from build123d import *

# Parameters (mm, degrees)
PAD_DEPTH          = 30
SKETCH001_R        = 1.698779
SKETCH001_R_2      = 1.697275
POCKET_DEPTH       = 137.607308
POCKET001_DEPTH    = 3.3
POCKET001_FACE8_W  = 30
POCKET001_FACE8_H  = 12.999695
POCKET001_FACE8_R  = 1.698779
POCKET002_DEPTH    = 0.2
POCKET002_FACE11_W = 30
POCKET002_FACE11_H = 13.000122
POCKET002_FACE11_R = 1.698779
POCKET003_DEPTH    = 0.2
POCKET003_FACE16_W = 30
POCKET003_FACE16_H = 13.005555
POCKET003_FACE16_R = 1.697275
POCKET004_DEPTH    = 0.2
POCKET004_FACE19_W = 30
POCKET004_FACE19_H = 13.004761
POCKET004_FACE19_R = 1.697275
POCKET005_DEPTH    = 0.2


with BuildPart() as part:
    # Sketch → Pad (new body)
    with BuildSketch(Plane.XZ.offset(-204.7)):
        Polygon((442.140533, 170.606308), (570.199951, 170.606308), (570.199951, 160.446457), (557.19519, 160.446457), (557.19519, 144.454102), (570.200745, 144.454102), (570.200745, 134.453659), (442.140106, 134.453659), (442.140106, 144.601944), (455.140228, 144.601944), (455.140228, 160.599991), (442.140533, 160.599991), align=None)
    extrude(amount=-PAD_DEPTH)

    # Sketch001 → Pocket (cut, through all)
    with BuildSketch(Plane.XY.offset(33)):
        with Locations((449.144109, 219.697878)):
            Circle(SKETCH001_R)
        with Locations((563.197394, 219.696552)):
            Circle(SKETCH001_R_2)
    extrude(amount=POCKET_DEPTH, mode=Mode.SUBTRACT)

    # Sketch002 → Pocket001 (cut)
    with BuildSketch(Plane.XY.offset(134.45)):
        Polygon((447.4586694554, 222.4277322113), (445.9354318133, 219.6021619882), (447.6208285856, 216.8702143825), (450.829463, 216.963837), (452.3527006421, 219.7894072231), (450.6673038698, 222.5213548287), align=None)
        Polygon((561.3429027745, 222.3136473905), (560.000239016, 219.3979392379), (561.8539844669, 216.7773042379), (565.0503936764, 217.0723773905), (566.393057435, 219.9880855431), (564.539311984, 222.6087205431), align=None)
    extrude(amount=POCKET001_DEPTH, mode=Mode.SUBTRACT)

    # Pocket001 Face8 → Pocket002 (cut)
    with BuildSketch(Plane(origin=(448.6283915528, 219.7000505045, 160.599991), x_dir=(0, -1, 0), z_dir=(0, 0, -1))):
        with Locations((5.05045e-05, -0.0119889472)):
            Rectangle(POCKET001_FACE8_W, POCKET001_FACE8_H)
        with Locations((0.0021725045, -0.5157174472)):
            Circle(POCKET001_FACE8_R, mode=Mode.SUBTRACT)
    extrude(amount=-POCKET002_DEPTH, mode=Mode.SUBTRACT)

    # Pocket002 Face11 → Pocket003 (cut)
    with BuildSketch(Plane(origin=(448.6281733748, 219.7000505028, 144.601944), x_dir=(0, 1, 0), z_dir=(0, 0, 1))):
        with Locations((-5.05028e-05, -0.0119936252)):
            Rectangle(POCKET002_FACE11_W, POCKET002_FACE11_H)
        with Locations((-0.0021725028, -0.5159356252)):
            Circle(POCKET002_FACE11_R, mode=Mode.SUBTRACT)
    extrude(amount=-POCKET003_DEPTH, mode=Mode.SUBTRACT)

    # Pocket003 Face16 → Pocket004 (cut)
    with BuildSketch(Plane(origin=(563.709854284, 219.7000818773, 144.454102), x_dir=(0, 1, 0), z_dir=(0, 0, 1))):
        with Locations((-8.18773e-05, 0.011886784)):
            Rectangle(POCKET003_FACE16_W, POCKET003_FACE16_H)
        with Locations((-0.0035298773, 0.512460284)):
            Circle(POCKET003_FACE16_R, mode=Mode.SUBTRACT)
    extrude(amount=-POCKET004_DEPTH, mode=Mode.SUBTRACT)

    # Pocket004 Face19 → Pocket005 (cut)
    with BuildSketch(Plane(origin=(563.7094485991, 219.7000818825, 160.446457), x_dir=(0, -1, 0), z_dir=(0, 0, -1))):
        with Locations((8.18825e-05, 0.0118780991)):
            Rectangle(POCKET004_FACE19_W, POCKET004_FACE19_H)
        with Locations((0.0035298825, 0.5120545991)):
            Circle(POCKET004_FACE19_R, mode=Mode.SUBTRACT)
    extrude(amount=-POCKET005_DEPTH, mode=Mode.SUBTRACT)


solid = part.part
Could you check a few things on this model? Use its own coordinates, in mm. A direction names the side the tool comes from. Give positions to 0.01 mm unless a question says otherwise; leave off trailing zeros. Order: outer loops, then holes, each group sorted by start corner. A loop starts at its lowest first (then second) coordinate and runs counter-clockwise, first axis right, second up.
1. For faces 1 (the flat face through (447, 220, 160.8)), 2 (the flat face through (446.708, 221.035, 136.079)), 3 (the flat face through (557.195, 219, 153)), 4 (the flat face through (505, 219, 170.606)), which set-ups out of +Z, -Z, +X, -X, +Y, -Y let a thin tool reach every point of the face, with its end or its side?
2. We'd pull the mould along Z, two halves only. Please class faces 5 (the flat face through (455.14, 220, 152)), 6 (the flat face through (565, 218, 137.75)), 7 (the flat face through (446.766, 218.255, 136.079)): pulls with the +Z half, pulls with the -Z half, needs draft (parallel to the pull), parting line crosses it, or undercut.
3. Suppose I cut it at A-A (y = 212). List the corners of the cut face in (x, z) for me.
4. I need wall thicknesses on L1, parallel to X at y = 219.5, z = 161.5; L2, parallel to X at y = 210, z = 159; L3, parallel to Z at x = 561, y = 216. Which ranges of each line are inside material? Lowest first, please.
5. Suppose I cut it at B-B (z = 151.5). List the corners of the cut face in (x, y) for me.
6. Will these pins go through, and if not, where does the flat tip stop? P1, Ø4.5, axis at x = 449.14, y = 219.7, coming from the -Z side; P2, Ø4, axis at y = 208.5, z = 150, coming from the +X side; P3, Ø6.5, axis at x = 564.5, y = 221.5, coming from the -Z side; P4, Ø5, axis at y = 225.5, z = 148.5, coming from the -X side.
Solved:
1. face 1: -X, +Y, -Y
1. face 2: -Z
1. face 3: +X, +Y, -Y
1. face 4: +Z, +X, -X, +Y, -Y
2. face 5: undercut
2. face 6: pulls with the -Z half
2. face 7: needs draft
3. outline: (442.14, 134.45) - (570.2, 134.45) - (570.2, 144.25) - (557.2, 144.25) - (557.2, 160.65) - (570.2, 160.65) - (570.2, 170.61) - (442.14, 170.61) - (442.14, 160.8) - (455.14, 160.8) - (455.14, 144.4) - (442.14, 144.4) - close
4. L1: x = 442.14 to 447.46, 450.83 to 561.51, 564.88 to 570.2
4. L2: x = 455.14 to 557.2
4. L3: z = 134.45 to 144.25, 160.65 to 170.61
5. outline: (455.14, 204.7) - (557.2, 204.7) - (557.2, 234.7) - (455.14, 234.7) - close
6. P1: stops at z = 137.75
6. P2: stops at x = 557.2
6. P3: stops at z = 134.45
6. P4: stops at x = 455.14
